Read the model definition and answer for the solid it produces. Units are mm, in the model's axes. A direction names the side the tool comes from. Coordinates: 2 decimals unless noted, no trailing zeros. Loops run counter-clockwise (first coordinate to the right, second up) from the corner with the lowest first, then second, coordinate; pieces in that order, holes last. Notation, with made-up numbers: (51, 75) - (77, 75) arc R22 ccw to (77, 104) - close; hole circle Ø7 at (-37.75, 20). An arc over 180 degrees is marked (long way). One line per item, written item: value. Start each with the question number.
from build123d import *

# Parameters (mm, degrees)
CHAMFER_2_SIZE           = 1.25
CHAMFER_2_SIZE2          = 0.334936491
CHAMFER_3_SIZE           = 1.25
CHAMFER_3_SIZE2          = 0.334936491
SKETCH_4_R               = 2
CUT_EXTRUDE_2_DEPTH      = 1
CUT_EXTRUDE_2_DEPTH_BACK = 8


with BuildPart() as part:
    # Эскиз2 → Повернуть2 (revolve)
    with BuildSketch(Plane.XY):
        Polygon((0, 0), (6.25, 0), (6.25, 3.5), (3, 3.5), (3, 7), (0, 7), align=None)
    revolve(axis=Axis((0, 7, 0), (0, -1, 0)))

    # Фаска2
    chamfer_2_edges = [part.edges().sort_by_distance(p)[0] for p in [
        (-6.25, 3.5, 0),
    ]]
    chamfer_2_side = [part.faces().sort_by_distance(p)[0] for p in [
        (-6.073223305, 3.5, 0),
    ]]
    chamfer(chamfer_2_edges, length=CHAMFER_2_SIZE, length2=CHAMFER_2_SIZE2, reference=chamfer_2_side[0])

    # Фаска3
    chamfer_3_edges = [part.edges().sort_by_distance(p)[0] for p in [
        (-6.25, 0, 0),
    ]]
    chamfer_3_side = [part.faces().sort_by_distance(p)[0] for p in [
        (0, 0, 0),
    ]]
    chamfer(chamfer_3_edges, length=CHAMFER_3_SIZE, length2=CHAMFER_3_SIZE2, reference=chamfer_3_side[0])

    # Эскиз4 → Вырез-Вытянуть2 (cut, two sides)
    with BuildSketch(Plane(origin=(0, 7, 0), x_dir=(1, 0, 0), z_dir=(0, 1, 0))) as cut_extrude_2_sk:
        Circle(SKETCH_4_R)
    extrude(amount=CUT_EXTRUDE_2_DEPTH, mode=Mode.SUBTRACT)
    extrude(cut_extrude_2_sk.sketch, amount=-CUT_EXTRUDE_2_DEPTH_BACK, mode=Mode.SUBTRACT)


solid = part.part
1) Section B-B, the plane x = 0 is taken. Determine the outline of the cut face in (y, z), and give its area (3 significant figures).
2) Determine the mould class of faces 3 (the flat face through (-2.2, 0, 0.1)), 4 (the cylindrical face through (5.96, 1.77, 1.88)), 5 (the cylindrical face through (0, 4, 2)) for opening direction X: released by +X, released by -X, zero draft, split by the parting line, or undercut.
3) Flat-ended cylindrical pins translate along their axes: P1, Ø4, axis at y = 5, z = -2.5, coming from the +X side; P2, Ø4, axis at y = 5, z = -3, coming from the -X side. Find the tip coordinate at first contact, or state that the pin passes through.
4) Section C-C, the plane y = 2.25 is taken. Determine the outline of the cut face in (x, z), and give its area (3 significant figures).
5) Section A-A, the plane z = 0 is taken. Determine the outline of the cut face in (x, y).
6) Straight lines are drawn through the part: L1, parallel to Z at x = 0, y = 5.25; L2, parallel to Z at x = 0, y = 3; L3, parallel to Y at x = -3.75, z = -1. For each, find the intervals that lie inside material, in ascending order.
7) Section D-D, the plane y = 5.75 is taken. Determine the outline of the cut face in (x, z).
8) For faces 1 (the flat face through (1, 7, -2)), 2 (the cylindrical face through (-3, 5, 0)), determine the directions among +Z, -Z, +X, -X, +Y, -Y from which every point of the face is accessible in a straight line to the end or side of a thin tool.
Answer below:
1. outline: (0, -5) - (0.33, -6.25) - (3.17, -6.25) - (3.5, -5) - (3.5, -3) - (7, -3) - (7, -2) - (0, -2) - close; (0, 2) - (7, 2) - (7, 3) - (3.5, 3) - (3.5, 5) - (3.17, 6.25) - (0.33, 6.25) - (0, 5) - close
1. area: 35.9 mm2
2. face 3: zero draft
2. face 4: split by the parting line
2. face 5: undercut
3. P1: x = 6.01
3. P2: x = -5.85
4. outline: circle Ø12.5 at (0, 0); hole circle Ø4 at (0, 0)
4. area: 110 mm2
5. outline: (-6.25, 0.33) - (-5, 0) - (-2, 0) - (-2, 7) - (-3, 7) - (-3, 3.5) - (-5, 3.5) - (-6.25, 3.17) - close; (2, 0) - (5, 0) - (6.25, 0.33) - (6.25, 3.17) - (5, 3.5) - (3, 3.5) - (3, 7) - (2, 7) - close
6. L1: -3 to -2, 2 to 3
6. L2: -6.25 to -2, 2 to 6.25
6. L3: 0 to 3.5
7. outline: circle Ø6 at (0, 0); hole circle Ø4 at (0, 0)
8. face 1: +Z, -Z, +X, -X, +Y
8. face 2: +Y
